Could you check a few things on this drawing? It's one solid part, dimensions in mm from its lowest x, y, z. Coordinates: 2 decimals unless noted, no trailing zeros. Write each loop counter-clockwise with the first axis right and the second up, starting at its lowest first coordinate (ties: lowest second). Pieces come first, ordered by that corner, then holes. Notation, with made-up numbers: M 15.25,77.25 L 69.25,77.25 A34 cw 69.25,108.25 Z; hole C 25.5,2.5 d4. An arc over 180 degrees is marked long. Use a Markdown table: item, result.
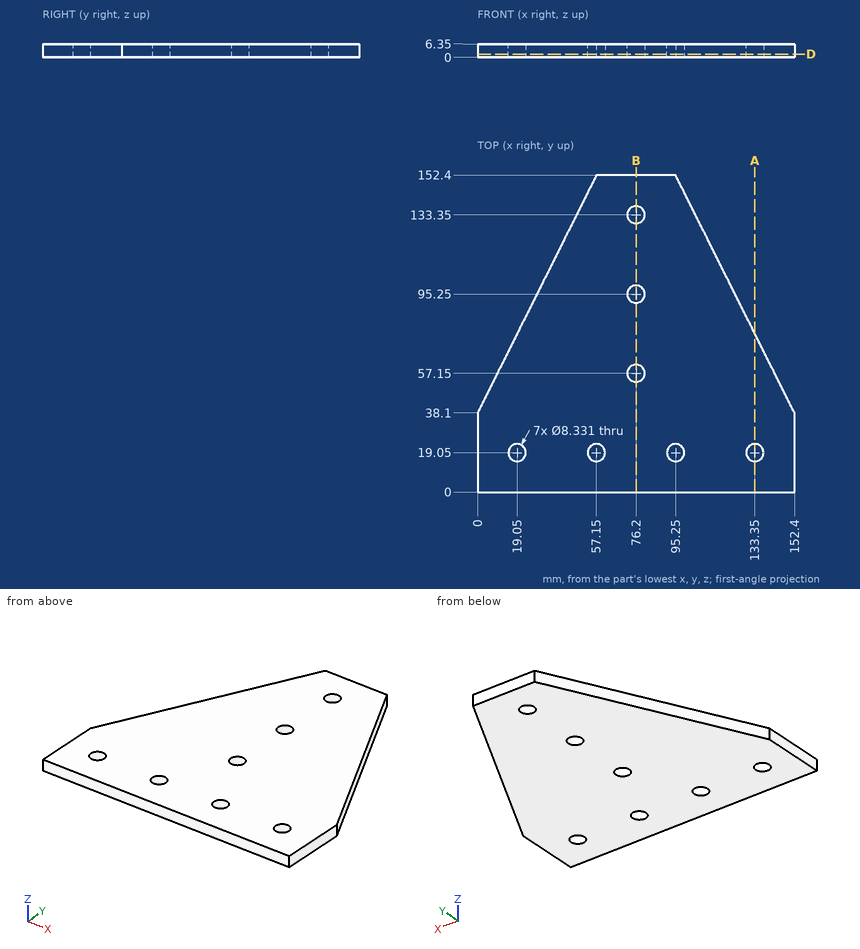
1. Will these pins go through, and if not, where does the flat tip stop? pin 1 Ø3 at (x, z) = (33.5, 3) entering from +Y; pin 2 Ø3 at (x, z) = (29, 5) entering from +Y.
Answers follow:
| item | result |
|---|---|
| pin 1 | stops at y = 108.1 |
| pin 2 | stops at y = 99.1 |
2. Suppose I cut it at D-D on z = 1.5. Write out the boundary of the cut face in (x, y).
Answers follow:
| item | result |
|---|---|
| outline | M 0,0 L 152.4,0 L 152.4,38.1 L 95.25,152.4 L 57.15,152.4 L 0,38.1 Z; hole C 19.05,19.05 d8.33; hole C 57.15,19.05 d8.33; hole C 76.2,57.15 d8.33; hole C 76.2,95.25 d8.33; hole C 76.2,133.35 d8.33; hole C 95.25,19.05 d8.33; hole C 133.35,19.05 d8.33 |
3. Suppose I cut it at A-A on x = 133.35. Write out the boundary of the cut face in (y, z), and give its area (3 significant figures).
Answers follow:
| item | result |
|---|---|
| outline | M 0,0 L 14.88,0 L 14.88,6.35 L 0,6.35 Z; M 23.22,0 L 76.2,0 L 76.2,6.35 L 23.22,6.35 Z |
| area | 431 mm2 |
4. I need wall thicknesses on probe 1 along Y at (x, z) = (77, 2.25); probe 2 along X at (y, z) = (55.5, 1.25) (1 decimal); probe 3 along Y at (x, z) = (21, 2.25). Which ranges of each line are inside material? Lowest first, please.
Answers follow:
| item | result |
|---|---|
| probe 1 | y = 0 to 53.06, 61.24 to 91.16, 99.34 to 129.26, 137.44 to 152.4 |
| probe 2 | x = 8.7 to 72.4, 80 to 143.7 |
| probe 3 | y = 0 to 15.37, 22.73 to 80.1 |
5. Suppose I cut it at B-B on x = 76.2. Write out the boundary of the cut face in (y, z).
Answers follow:
| item | result |
|---|---|
| outline | M 0,0 L 52.98,0 L 52.98,6.35 L 0,6.35 Z; M 61.32,0 L 91.08,0 L 91.08,6.35 L 61.32,6.35 Z; M 99.42,0 L 129.18,0 L 129.18,6.35 L 99.42,6.35 Z; M 137.52,0 L 152.4,0 L 152.4,6.35 L 137.52,6.35 Z |
